Design review of the part built by this model. Coordinates are the model's own, in mm. Face numbers are marked on the shaded views. Coordinates: 2 decimals unless noted, no trailing zeros. Write each loop counter-clockwise with the first axis right and the second up, starting at its lowest first coordinate (ties: lowest second). Pieces come first, ordered by that corner, then holes.
Q1. To check wall thickness, follow probe 1 along Y at (x, z) = (0, 0.85); probe 2 along X at (y, z) = (5, 0.2); probe 3 along X at (y, z) = (-12, 1.45). State the ranges of each line that lie inside material, in increasing order.
Q2. Add section D-D, the plane y = -3. Give the boundary of the cut face in (x, z), plus the area to 3 significant figures.
Q3. Add section C-C, the plane y = -6. Give the boundary of the cut face in (x, z).
Q4. The part is to be moulded in two halves that separate along Y. For the marked faces 1, 2 and 3, say which applies: +Y half, -Y half, draft (parallel to the pull), parting line (faces both ways), or undercut.
Q5. Clearance check with a flat-ended pin moving along its axis: pin 1 Ø1.5 at (x, z) = (-6.5, 1.5) entering from +Y. State where the tip first meets the part, or that it passes through.
Q6. Add section A-A, the plane y = 0. Give the boundary of the cut face in (x, z).
Q7. Add section B-B, the plane x = 0. Give the boundary of the cut face in (y, z).
from build123d import *

# Parameters (mm, degrees)
SKETCH_1_R          = 15
SKETCH_1_R_2        = 2
SKETCH_1_R_3        = 5
EXTRUDE_1_DEPTH     = 7
SKETCH_2_R          = 8
SKETCH_2_R_2        = 5
EXTRUDE_2_DEPTH     = 70
SKETCH_3_R          = 2.5
CUT_EXTRUDE_1_DEPTH = 10
CUT_EXTRUDE_START   = -4
SKETCH_4_R          = 18.074037985
SKETCH_4_R_2        = 8
CUT_EXTRUDE_2_DEPTH = 4
SKETCH_5_R          = 8.2
CUT_EXTRUDE_3_DEPTH = 90


with BuildPart() as part:
    # 草图1 → 凸台-拉伸1 (new body)
    with BuildSketch(Plane.XY):
        Circle(SKETCH_1_R)
        with Locations((0, 12)):
            Circle(SKETCH_1_R_2, mode=Mode.SUBTRACT)
        with Locations((10.392304845, 6)):
            Circle(SKETCH_1_R_2, mode=Mode.SUBTRACT)
        with Locations((10.392304845, -6)):
            Circle(SKETCH_1_R_2, mode=Mode.SUBTRACT)
        with Locations((0, -12)):
            Circle(SKETCH_1_R_2, mode=Mode.SUBTRACT)
        with Locations((-10.392304845, -6)):
            Circle(SKETCH_1_R_2, mode=Mode.SUBTRACT)
        with Locations((-10.392304845, 6)):
            Circle(SKETCH_1_R_2, mode=Mode.SUBTRACT)
        with Locations((-6, 10.392304845)):
            Circle(SKETCH_1_R_2, mode=Mode.SUBTRACT)
        with Locations((12, 0)):
            Circle(SKETCH_1_R_2, mode=Mode.SUBTRACT)
        with Locations((-6, -10.392304845)):
            Circle(SKETCH_1_R_2, mode=Mode.SUBTRACT)
        Circle(SKETCH_1_R_3, mode=Mode.SUBTRACT)
    extrude(amount=EXTRUDE_1_DEPTH)

    # 草图2 → 凸台-拉伸2 (add)
    with BuildSketch(Plane.XY.offset(7)):
        Circle(SKETCH_2_R)
        Circle(SKETCH_2_R_2, mode=Mode.SUBTRACT)
    extrude(amount=EXTRUDE_2_DEPTH)

    # 草图3 → 切除-拉伸1 (cut)
    with BuildSketch(Plane(origin=(0, 0, 0), x_dir=(1, 0, 0), z_dir=(0, 1, 0))):
        with Locations(Location((0.676832819, -59, 0), (0, 0, 270))):
            Circle(SKETCH_3_R)
    extrude(amount=-CUT_EXTRUDE_1_DEPTH, mode=Mode.SUBTRACT)

    # 草图4 → 切除-拉伸2 (cut)
    with BuildSketch(Plane.XY.offset(7).offset(CUT_EXTRUDE_START)):
        Circle(SKETCH_4_R)
        Circle(SKETCH_4_R_2, mode=Mode.SUBTRACT)
    extrude(amount=CUT_EXTRUDE_2_DEPTH, mode=Mode.SUBTRACT)

    # 草图5 → 切除-拉伸3 (cut)
    with BuildSketch(Plane.XY.offset(77)):
        Circle(SKETCH_5_R)
    extrude(amount=-CUT_EXTRUDE_3_DEPTH, mode=Mode.SUBTRACT)


solid = part.part
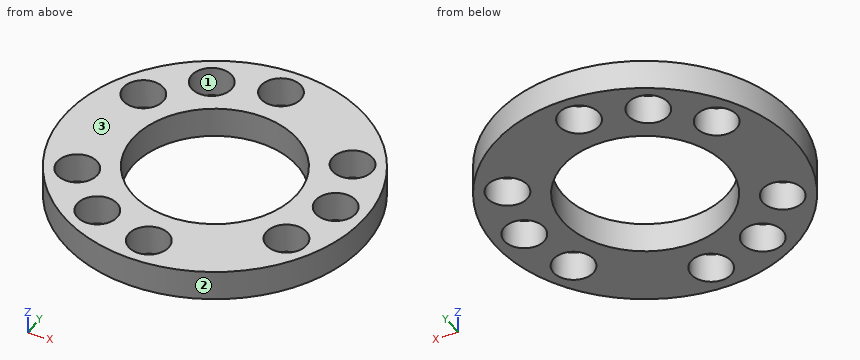
Here are the results:
1. probe 1: y = -15 to -14, -10 to -8.2, 8.2 to 10, 14 to 15
1. probe 2: x = -14.14 to -12.12, -8.66 to -6.5, 6.5 to 8.66, 12.12 to 14.14
1. probe 3: x = -9 to -7.19, -4.81 to -2, 2 to 9
2. outline: (-14.7, 0) - (-7.63, 0) - (-7.63, 3) - (-14.7, 3) - close; (7.63, 0) - (14.7, 0) - (14.7, 3) - (7.63, 3) - close
2. area: 42.4 mm2
3. outline: (-13.75, 0) - (-12.39, 0) - (-12.39, 3) - (-13.75, 3) - close; (-8.39, 0) - (-5.59, 0) - (-5.59, 3) - (-8.39, 3) - close; (5.59, 0) - (8.39, 0) - (8.39, 3) - (5.59, 3) - close; (12.39, 0) - (13.75, 0) - (13.75, 3) - (12.39, 3) - close
4. face 1: undercut
4. face 2: parting line
4. face 3: draft
5. pin 1: stops at y = 13.85
6. outline: (-15, 0) - (-8.2, 0) - (-8.2, 3) - (-15, 3) - close; (8.2, 0) - (10, 0) - (10, 3) - (8.2, 3) - close; (14, 0) - (15, 0) - (15, 3) - (14, 3) - close
7. outline: (-15, 0) - (-14, 0) - (-14, 3) - (-15, 3) - close; (-10, 0) - (-8.2, 0) - (-8.2, 3) - (-10, 3) - close; (8.2, 0) - (10, 0) - (10, 3) - (8.2, 3) - close; (14, 0) - (15, 0) - (15, 3) - (14, 3) - close
